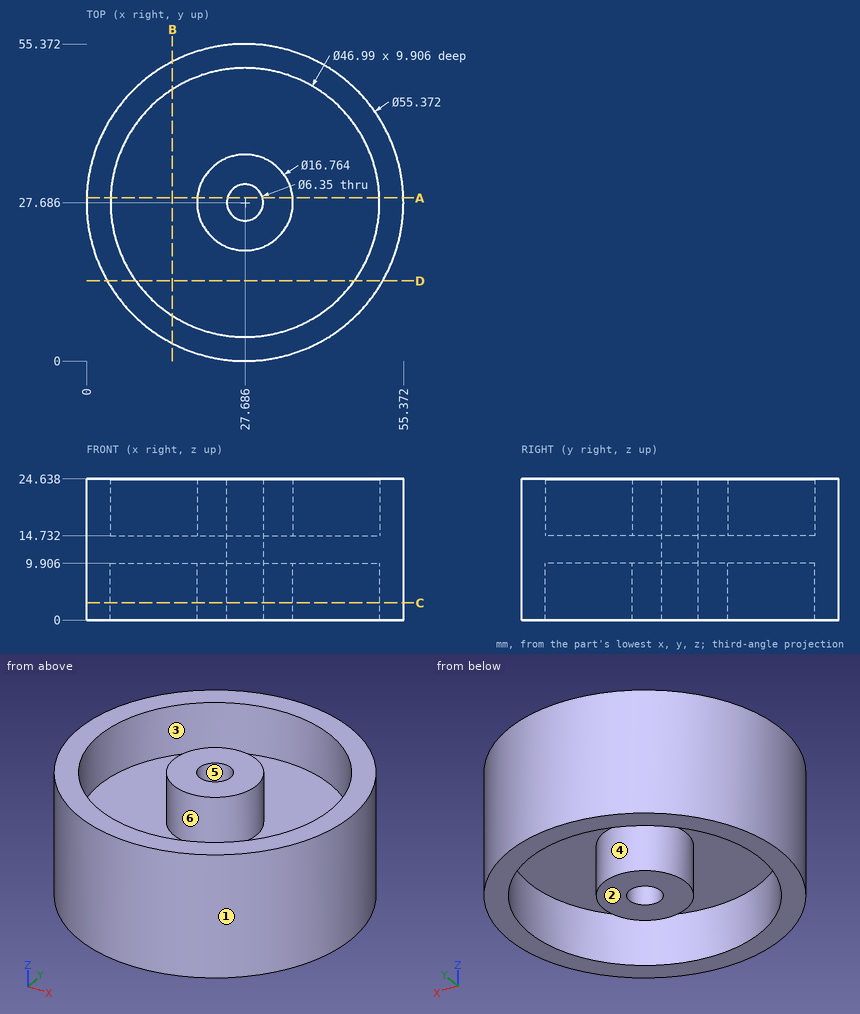
Drawing for the job (mm, zero at the part's lowest x, y, z). A direction names the side the tool comes from. Round coordinates to 2 decimals unless told otherwise and drop trailing zeros. Loops run counter-clockwise (first coordinate to the right, second up) from the corner with the lowest first, then second, coordinate; pieces in that order, holes last. Notation, with made-up numbers: (17, 12.5) -> (49, 12.5) arc R14 cw to (49, 38.5) -> close; hole circle Ø11 at (62.5, 36.5). An arc over 180 degrees is marked (long way). Use one line per item in the form item = value. Start each with the question number.
Item 1: Tool access for the marked faces 4, 5 and 6: list every direction of +Z, -Z, +X, -X, +Y, -Y with a clear straight run to the whole face (end or side of a thin tool).
Item 2: Band-saw the part on A-A (y = 28.5). List the corners of the cut face in (x, z), plus the area to 3 significant figures.
Item 3: Band-saw the part on C-C (z = 3). List the corners of the cut face in (x, y) (3 decimals).
Item 4: Drop flat-ended pins along their axis: pin 1 Ø1 at (x, z) = (15, 15.5) entering from -Y; pin 2 Ø3 at (x, y) = (39, 19) entering from +Z; pin 3 Ø10 at (y, z) = (45.5, 5.5) entering from -X; pin 4 Ø5.5 at (x, y) = (27.686, 27.686) entering from +Z. Give the stop position or say it passes through.
Item 5: Two-plate mould, pull along X, no slides. Class the marked faces 1, 2 and 3: released by +X, released by -X, zero draft, split by the parting line, or undercut.
Item 6: Band-saw the part on D-D (y = 14). List the corners of the cut face in (x, z), plus the area to 3 significant figures.
Item 7: Band-saw the part on B-B (x = 15). List the corners of the cut face in (y, z), plus the area to 3 significant figures.
Item 8: Drill centre lines: line 1 along Y through (x, z) = (35, 5.25); line 2 along Y through (x, z) = (24, 18.75); line 3 along X through (y, z) = (23.5, 23). Where is each one in solid material? Low to high.
Data:
q1.face_4 = -Z
q1.face_5 = +Z, -Z
q1.face_6 = +Z
q2.outline = (0.01, 0) -> (4.21, 0) -> (4.21, 9.91) -> (19.34, 9.91) -> (19.34, 0) -> (24.62, 0) -> (24.62, 24.64) -> (19.34, 24.64) -> (19.34, 14.73) -> (4.21, 14.73) -> (4.21, 24.64) -> (0.01, 24.64) -> close; (30.75, 0) -> (36.03, 0) -> (36.03, 9.91) -> (51.17, 9.91) -> (51.17, 0) -> (55.36, 0) -> (55.36, 24.64) -> (51.17, 24.64) -> (51.17, 14.73) -> (36.03, 14.73) -> (36.03, 24.64) -> (30.75, 24.64) -> close
q2.area = 613 mm^2
q3.outline = circle Ø55.372 at (27.686, 27.686); circle Ø16.764 at (27.686, 27.686); hole circle Ø46.99 at (27.686, 27.686); hole circle Ø6.35 at (27.686, 27.686)
q4.pin_1 = 2.83
q4.pin_2 = 14.73
q4.pin_3 = 3.14
q4.pin_4 = through
q5.face_1 = split by the parting line
q5.face_2 = zero draft
q5.face_3 = undercut
q6.outline = (3.62, 0) -> (8.59, 0) -> (8.59, 9.91) -> (46.78, 9.91) -> (46.78, 0) -> (51.75, 0) -> (51.75, 24.64) -> (46.78, 24.64) -> (46.78, 14.73) -> (8.59, 14.73) -> (8.59, 24.64) -> (3.62, 24.64) -> close
q6.area = 429 mm^2
q7.outline = (3.08, 0) -> (7.91, 0) -> (7.91, 9.91) -> (47.46, 9.91) -> (47.46, 0) -> (52.29, 0) -> (52.29, 24.64) -> (47.46, 24.64) -> (47.46, 14.73) -> (7.91, 14.73) -> (7.91, 24.64) -> (3.08, 24.64) -> close
q7.area = 429 mm^2
q8.line_1 = 0.98 to 5.36, 23.59 to 31.78, 50.01 to 54.39
q8.line_2 = 0.25 to 4.48, 20.16 to 35.21, 50.89 to 55.13
q8.line_3 = 0.32 to 4.57, 20.42 to 34.95, 50.81 to 55.05
